Geometry check sheet. Reference: the model listing, model coordinates, mm. A direction names the side the tool comes from. Round coordinates to 2 decimals unless told otherwise and drop trailing zeros. Loops run counter-clockwise (first coordinate to the right, second up) from the corner with the lowest first, then second, coordinate; pieces in that order, holes last. Notation, with made-up numbers: (31, 54.25) - (68, 54.25) arc R21 ccw to (68, 65.25) - close; hole circle Ø8 at (-22, -4.75). An arc over 180 degrees is marked (long way). Answer as CSV lines item,"result". Start each with the question number.
1) Depth check by flat-ended pin: P1, Ø4, axis at x = -17, y = -1.5, coming from the +Z side; P2, Ø3, axis at x = -13, z = 2, coming from the -Y side; P3, Ø10, axis at x = -5.5, z = 8, coming from the +Y side; P4, Ø6.5, axis at x = -33, z = 0, coming from the +Y side. Enter the tip coordinate at first touch or a pass-through.
2) Cross-section at A-A on x = -3.5. Record the boundary of the cut face in (y, z), and give its area (3 significant figures).
3) Cross-section at D-D on x = -33. Record the boundary of the cut face in (y, z), and give its area (3 significant figures).
4) Draft check along Z on faces 3 (the flat face through (0, 5, 5)), 4 (the conical face through (-27.1, 0.33, -1.04)), 5 (the cylindrical face through (-20.469, 9.759, -5.076)). Enter one of: released by +Z, released by -Z, zero draft, split by the parting line, or undercut.
5) Thickness scan on line 1 along Y through (x, z) = (-16, 0); line 2 along Y through (x, z) = (-20, 4.5); line 3 along Z through (x, y) = (-30, 8.25). Record the ranges inside material, lowest first.
6) Access from +Z, -Z, +X, -X, +Y, -Y to the whole of each face (thin tool, end or side, straight path). Record for faces 1 (the cylindrical face through (-12.17, 1.88, 5.96)), 2 (the cylindrical face through (-29.034, -0.154, -0.521)).
7) Cross-section at B-B on y = 9. Record the boundary of the cut face in (x, z).
8) Cross-section at C-C on z = -7.75. Record the boundary of the cut face in (x, y), and give its area (3 significant figures).
from build123d import *

# Parameters (mm, degrees)
M14X1_5_1_D              = 12.5
M14X1_5_1_DEPTH          = 24
M14X1_5_1_TIP            = 3.755378869
CUT_EXTRUDE_1_DEPTH      = 45.788391353
CUT_EXTRUDE_1_DEPTH_BACK = 45.788391353
SKETCH_4_R               = 4


with BuildPart() as part:
    # 草图1 → 旋转1 (revolve)
    with BuildSketch(Plane.XY, mode=Mode.PRIVATE) as revolve_1_sk:
        with BuildLine():
            Line((0, 0), (0, 11))
            Line((0, 11), (-40.373066959, 11))
            ThreePointArc((-40.373066959, 11), (-41.591066388, 5.559831632), (-42, 0))
            Line((-42, 0), (0, 0))
        make_face()
    revolve(revolve_1_sk.sketch.rotate(Axis((0, 0, 0), (-1, 0, 0)), 90), axis=Axis((0, 0, 0), (-1, 0, 0)))

    # M14X1.5 螺纹孔的螺纹孔钻头1
    with Locations(Plane(origin=(0, 0, 0), x_dir=(0, 0, -1), z_dir=(1, 0, 0))):
        with Locations((0, 0)):
            Hole(M14X1_5_1_D / 2, depth=M14X1_5_1_DEPTH)
            with Locations((0, 0, -(M14X1_5_1_DEPTH + M14X1_5_1_TIP / 2))):  # 118° drill point
                Cone(0, M14X1_5_1_D / 2, M14X1_5_1_TIP, mode=Mode.SUBTRACT)

    # 草图4 → 切除-拉伸1 (cut, two sides: drawn at the far end of the back side and taken through both)
    with BuildSketch(Plane(origin=(0, 0, 0), x_dir=(1, 0, 0), z_dir=(0, 1, 0)).offset(-CUT_EXTRUDE_1_DEPTH_BACK)):
        with Locations(Location((-33, 0, 0), (0, 0, 270))):
            Circle(SKETCH_4_R)
    extrude(amount=CUT_EXTRUDE_1_DEPTH + CUT_EXTRUDE_1_DEPTH_BACK, mode=Mode.SUBTRACT)


solid = part.part
Answer block:
1,P1,"stops at z = 11"
1,P2,"stops at y = -10.99"
1,P3,"stops at y = 10.58"
1,P4,"passes through"
2,outline,"circle Ø22 at (0, 0); hole circle Ø12.5 at (0, 0)"
2,area,"257 mm^2"
3,outline,"(-10.25, -4) arc R11 ccw to (10.25, -4) - close; (-10.25, 4) - (10.25, 4) arc R11 ccw to start"
3,area,"208 mm^2"
4,face 3,"zero draft"
4,face 4,"undercut"
4,face 5,"split by the parting line"
5,line 1,"y = -11 to -6.25, 6.25 to 11"
5,line 2,"y = -10.04 to -4.34, 4.34 to 10.04"
5,line 3,"z = -7.28 to -2.65, 2.65 to 7.28"
6,face 1,"+X"
6,face 2,"+Y, -Y"
7,outline,"(-40.37, -6.32) - (0, -6.32) - (0, 6.32) - (-40.37, 6.32) arc R36.92 ccw to start; hole circle Ø8 at (-33, 0)"
8,outline,"(-40.37, -7.81) - (0, -7.81) - (0, 7.81) - (-40.37, 7.81) arc R37.2 ccw to start"
8,area,"639 mm^2"
